Can you work these out from the model? Positions are in its coordinate system, mm. A direction names the side the tool comes from. Round coordinates to 2 decimals unless told otherwise and drop trailing zeros. Loops run counter-clockwise (first coordinate to the right, second up) from the corner with the lowest first, then second, coordinate; pieces in that order, holes last. Notation, with made-up numbers: (-28.75, 85.25) -> (-14.75, 85.25) arc R18 ccw to (-14.75, 107.25) -> close; hole circle Ø5 at (48.5, 11). An arc over 180 degrees is marked (long way). Write each question's results on one line, items separated by ' | '.
Autodesk Inventor part; units mm, degrees
ref_plane "YZ Plane" through (0, 0, 0) normal (1, 0, 0) x (0, 1, 0)
ref_plane "XZ Plane" through (0, 0, 0) normal (0, 1, 0) x (-1, 0, 0)
ref_plane "XY Plane" through (0, 0, 0) normal (0, 0, 1) x (1, 0, 0)
sketch "スケッチ1" plane through (0, 0, 0) normal (0, 0, 1) x (1, 0, 0)
  line L0 (-20, -2.5) -> (20, -2.5)
  line L1 (20, -2.5) -> (20, 2.5)
  line L2 (-20, 2.5) -> (-20, -2.5)
  line L3 (-20, -2.5) -> (20, 2.5) construction
  line L4 (20, -2.5) -> (-20, 2.5) construction
  line L5 (-10, 2.5) -> (10, 2.5)
  line L6 (10, 2.5) -> (10, 52.5)
  line L7 (10, 52.5) -> (-10, 52.5)
  line L8 (-10, 52.5) -> (-10, 2.5)
  line L9 (-10, 2.5) -> (10, 52.5) construction
  line L10 (10, 2.5) -> (-10, 52.5) construction
  line L11 (20, 2.5) -> (10, 2.5)
  line L12 (-10, 2.5) -> (-20, 2.5)
  line L13 (0, 52.5) -> (0, -2.5)
  point P0 (0, 0)
  point P1 (0, 27.5)
  point P2 (0, 27.5)
  point P3 (0, 0)
  dimension "d0" = 20
  dimension "d1" = 50
  dimension "d2" = 5
  dimension "d3" = 10
extrude "押し出し1" add sketch "スケッチ1" along normal mid plane 210 contours L2 L12 L5 L13 L0 | L5 L8 L7 L13
sketch "スケッチ8" plane through (-10, 2.5, 105) normal (-1, 0, 0) x (0, 0, 1)
  line L0 (-210, 50) -> (0, 50)
  line L1 (-33.61, 50) -> (0, 2)
  line L2 (0, -5) -> (0, 50)
  line L3 (-210, 0) -> (0, 0)
  point P0 (-105, -2.5)
  dimension "d60" = 2
  dimension "d68" = 145
extrude "押し出し5" cut sketch "スケッチ8" against normal blind 210
sketch "スケッチ9" plane through (-10, 2.5, -105) normal (-1, 0, 0) x (0, 0, 1)
  circle A0 centre (158, 41) radius 6.05
  line L0 (210, 2) -> (210, 0)
  line L1 (0, 0) -> (210, 0)
  point P0 (105, -2.5)
  dimension "d63" = 12.1
  dimension "d64" = 52
  dimension "d65" = 41
extrude "押し出し6" cut sketch "スケッチ9" against normal blind 210
sketch "スケッチ10" plane through (-20, 2.5, 105) normal (0, 1, 0) x (1, 0, 0)
  line L0 (0, 210) -> (0, 0)
  line L1 (10, 0) -> (0, 0)
  line L2 (0, 210) -> (10, 210)
  point P0 (20, 105)
  point P1 (5, 5)
  point P2 (5, 79.86)
  point P3 (5, 96.483)
  point P4 (5, 205)
  dimension "d69" = 5
  dimension "d70" = 5
  dimension "d71" = 74.86
  dimension "d72" = 16.623
  dimension "d73" = 5
hole "穴5" at (-15, 2.5, -100) at (-15, 2.5, 100) direction (0, -1, 0) diameter 3.2 end through all
hole "穴6" at (-15, 2.5, 25.14) at (-15, 2.5, 8.517) direction (0, -1, 0) diameter 5.2 end through all
properties part number "s_base4"
1. If we section it at A-A (z = 25.14): List the corners of the cut face in (x, y) for me.
Final values:
outline: (-20, -2.5) -> (-17.6, -2.5) -> (-17.6, 2.5) -> (-20, 2.5) -> close; (-12.4, -2.5) -> (0, -2.5) -> (0, 52.5) -> (-10, 52.5) -> (-10, 2.5) -> (-12.4, 2.5) -> close
2. If we section it at D-D (z = -44.5): List the corners of the cut face in (x, y) for me, then the cut area to 3 significant figures.
Final values:
outline: (-20, -2.5) -> (0, -2.5) -> (0, 52.5) -> (-10, 52.5) -> (-10, 2.5) -> (-20, 2.5) -> close | area: 600 mm2
3. If we section it at C-C (y = 43.5): List the corners of the cut face in (x, z) for me.
Final values:
outline: (-10, -105) -> (0, -105) -> (0, 46.95) -> (-10, 46.95) -> close; (-10, 59.05) -> (0, 59.05) -> (0, 77.69) -> (-10, 77.69) -> close
4. Please list where these lines run through material, in increasing order: line 1 (Z direction, x = -15, y = -0.65); line 2 (X direction, y = -1.15, z = -100); line 3 (Y direction, x = -6.5, z = 53). Write a range as from..to.
Final values:
line 1: -105..-101.6, -98.4..5.92, 11.12..22.54, 27.74..98.4, 101.6..105 | line 2: -20..-16.6, -13.4..0 | line 3: -2.5..37.45, 49.55..52.5
5. Will these pins go through, and if not, where does the flat tip stop? pin 1 (10 mm diameter, centred on y = 11.5, z = -38.5, fed in from -X); pin 2 (5 mm diameter, centred on x = -16.5, z = -3, fed in from +Y); pin 3 (11 mm diameter, centred on y = 43.5, z = 53, fed in from -X); pin 4 (10 mm diameter, centred on x = -3, y = 35, fed in from +Z).
Final values:
pin 1: x = -10 | pin 2: y = 2.5 | pin 3: through | pin 4: z = 87.14
6. We'd pull the mould along Z, two halves only. Please class faces 3 (the face through (-6, 25, -105)), 4 (the face through (-13.418, -0.035, 23.077)), 5 (the face through (-10, -2.5, -1)), 6 (the face through (-10, 0, 105)): pulls with the +Z half, pulls with the -Z half, needs draft (parallel to the pull), parting line crosses it, or undercut.
Final values:
face 3: pulls with the -Z half | face 4: undercut | face 5: needs draft | face 6: pulls with the +Z half
7. On a 3-axis mill with a long thin cutter (end or side, diameter ignored), from which of +Z, -Z, +X, -X, +Y, -Y can I reach the whole of each face in a straight line? I mean faces 1 (the face through (-5.07, 28.836, 87.96)), 2 (the face through (-15, 2.5, -1)). Say none if no direction works.
Final values:
face 1: +Z, +X, -X, +Y | face 2: +Z, -Z, -X, +Y
8. If we section it at B-B (x = -5): List the corners of the cut face in (y, z) for me, then the cut area to 3 significant figures.
Final values:
outline: (-2.5, -105) -> (52.5, -105) -> (52.5, 71.39) -> (4.5, 105) -> (-2.5, 105) -> close; hole circle Ø12.1 at (43.5, 53) | area: 10,600 mm2
